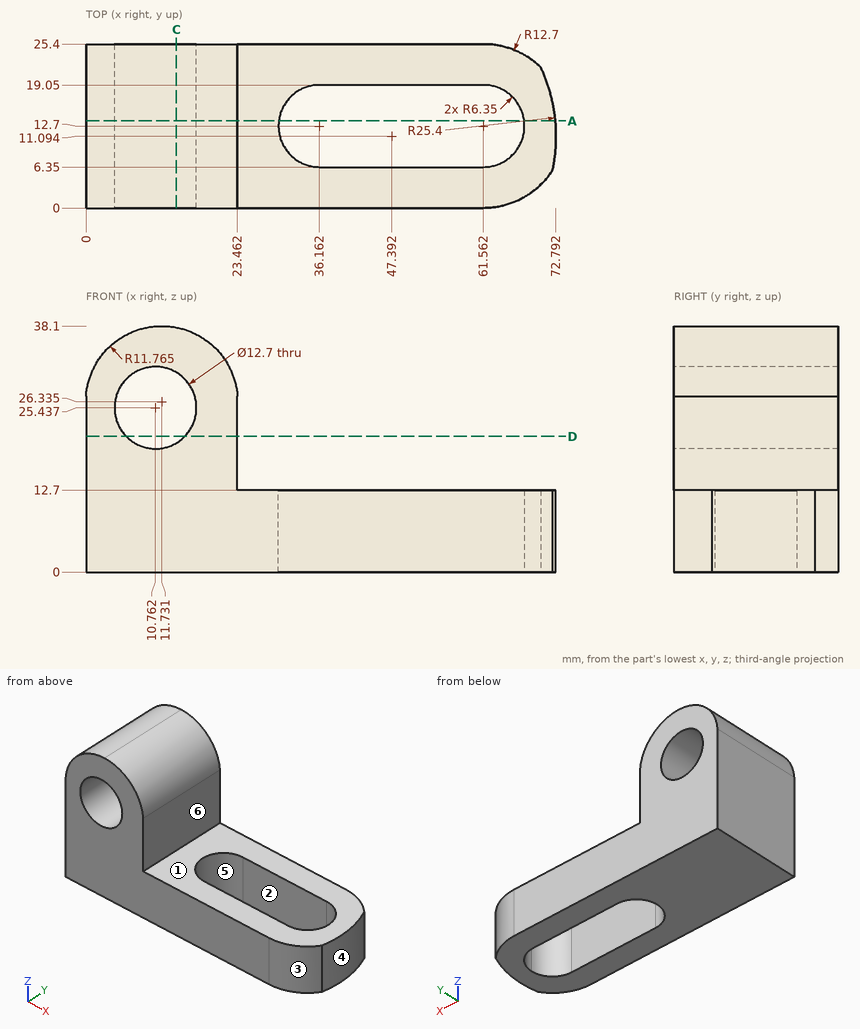
Check sheet for the drawn part. Datum: minimum x, y, z corner. Units: mm. A direction names the side the tool comes from. Give positions to 0.01 mm unless a question says otherwise; leave off trailing zeros. Write each loop counter-clockwise with the first axis right and the second up, starting at its lowest first coordinate (ties: lowest second). Pieces come first, ordered by that corner, then holes.
(1) Cross-section at D-D (z = 21). Enter the section's corners in (x, y) (1 decimal), plus the area to 3 significant figures.
(2) Mould release check, pull along X, two halves, no side actions. Record for the marked faces 1, 2 and 3: +X half, -X half, draft (parallel to the pull), parting line (faces both ways), or undercut.
(3) Access from +Z, -Z, +X, -X, +Y, -Y to the whole of each face (thin tool, end or side, straight path). Record for the marked faces 4, 5 and 6.
(4) Gauge pin test, flat ends, axial feed: pin 1 (10 mm diameter, centred on y = 14, z = 4.5, fed in from -X); pin 2 (7.5 mm diameter, centred on x = 52, y = 13, fed in from +Z); pin 3 (3 mm diameter, centred on x = 61, y = 20, fed in from +Z); pin 4 (4.5 mm diameter, centred on y = 15, z = 21, fed in from +X). Record the tip position at first contact, or that the pin passes through.
(5) Cross-section at A-A (y = 13.5). State how many separate pieces and enclosed holes the cut face has, plus the area to 3 significant figures.
(6) Material ranges on line 1 (Z direction, x = 23.5, y = 15.25); line 2 (X direction, y = 6.25, z = 15); line 3 (Z direction, x = 5, y = 14.5) (1 decimal), recorded low to high.
(7) Cross-section at C-C (x = 14). Enter the section's corners in (y, z) (1 decimal), plus the area to 3 significant figures.
Worked out:
1. outline: (0, 0) - (6.2, 0) - (6.2, 25.4) - (0, 25.4) - close; (15.3, 0) - (23.5, 0) - (23.5, 25.4) - (15.3, 25.4) - close
1. area: 365 mm2
2. face 1: draft
2. face 2: undercut
2. face 3: +X half
3. face 4: +Z, -Z, +X
3. face 5: +Z, -Z
3. face 6: +Z, +X, +Y, -Y
4. pin 1: stops at x = 0
4. pin 2: passes through
4. pin 3: stops at z = 12.7
4. pin 4: stops at x = 23.46
5. separate pieces: 2
5. enclosed holes: 1
5. area: 851 mm2
6. line 1: z = 0 to 12.7
6. line 2: x = 0 to 23.46
6. line 3: z = 0 to 22.8, 28.1 to 36
7. outline: (0, 0) - (25.4, 0) - (25.4, 20) - (0, 20) - close; (0, 30.9) - (25.4, 30.9) - (25.4, 37.9) - (0, 37.9) - close
7. area: 685 mm2
